from build123d import *

# Parameters (mm, degrees)
BOSS_EXTRUDE1_DEPTH = 8
SKETCH2_R           = 26
SKETCH2_R_2         = 22.5
EXTRUDE_THIN1_DEPTH = 50
SKETCH3_R           = 24.5
SKETCH3_R_2         = 22.5
EXTRUDE_THIN2_DEPTH = 40


with BuildPart() as part:
    # Sketch1 → Boss-Extrude1 (new body)
    with BuildSketch(Plane(origin=(0, 0, 0), x_dir=(1, 0, 0), z_dir=(0, 1, 0))):
        with BuildLine():
            ThreePointArc((-7.74066092, -30.276140252), (0, -31.25), (7.74066092, -30.276140252))
            ThreePointArc((7.74066092, -30.276140252), (32.571933158, -26.108732409), (57.750443262, -26.153431792))
            ThreePointArc((57.750443262, -26.153431792), (86.25, 0), (57.750443262, 26.153431792))
            ThreePointArc((57.750443262, 26.153431792), (32.571933158, 26.108732409), (7.74066092, 30.276140252))
            ThreePointArc((7.74066092, 30.276140252), (0, 31.25), (-7.74066092, 30.276140252))
            ThreePointArc((-7.74066092, 30.276140252), (-32.571933158, 26.108732409), (-57.750443262, 26.153431792))
            ThreePointArc((-57.750443262, 26.153431792), (-86.25, 0), (-57.750443262, -26.153431792))
            ThreePointArc((-57.750443262, -26.153431792), (-32.571933158, -26.108732409), (-7.74066092, -30.276140252))
        make_face()
    extrude(amount=BOSS_EXTRUDE1_DEPTH)

    # Sketch2 → Extrude-Thin1 (add)
    with BuildSketch(Plane(origin=(0, 8, 0), x_dir=(1, 0, 0), z_dir=(0, 1, 0))):
        Circle(SKETCH2_R)
        Circle(SKETCH2_R_2, mode=Mode.SUBTRACT)
    extrude(amount=EXTRUDE_THIN1_DEPTH)

    # Sketch3 → Extrude-Thin2 (add)
    # profile 1 of 2: a face of its own
    with BuildSketch(Plane.XZ):
        with Locations((-60, 0)):
            Circle(SKETCH3_R)
        with Locations((-60, 0)):
            Circle(SKETCH3_R_2, mode=Mode.SUBTRACT)
    # profile 2 of 2: a face of its own
    with BuildSketch(Plane.XZ):
        with Locations((60, 0)):
            Circle(SKETCH3_R)
        with Locations((60, 0)):
            Circle(SKETCH3_R_2, mode=Mode.SUBTRACT)
    extrude(amount=EXTRUDE_THIN2_DEPTH)


solid = part.part
Read the model definition and answer for the solid it produces. Units are mm, in the model's axes. A direction names the side the tool comes from. Round coordinates to 2 decimals unless told otherwise and drop trailing zeros. Loops run counter-clockwise (first coordinate to the right, second up) from the corner with the lowest first, then second, coordinate; pieces in that order, holes last.
Q1. Section C-C on z = -2 is taken. Write down the section's boundary in (x, y), and give its area (3 significant figures).
Q2. Which of the six approach directions +Z, -Z, +X, -X, +Y, -Y give full straight-line access (tool end or side, diameter ignored) to faces 1 (the face through (-60, 0, 0)), 2 (the face through (32.92, 3.94, -26.08)), 3 (the face through (0, 8, 0))?
Q3. Each of these flat-tipped pins is pushed along its axis until it touches: pin 1 (10 mm diameter, centred on x = -4, z = -6.5, fed in from +Y); pin 2 (1 mm diameter, centred on y = 2, z = 8, fed in from +X); pin 3 (1 mm diameter, centred on x = -9.5, z = 23.5, fed in from -Y). Where does it stop, or does it pass through?
Q4. Determine the mould class of faces 4 (the face through (0.11, 3.94, -31.25)), 5 (the face through (10.382, 32.65, 19.961)), 6 (the face through (-32.92, 3.94, 26.08)) for opening direction Z: released by +Z, released by -Z, zero draft, split by the parting line, or undercut.
Q5. Consider probe 1 along X at (y, z) = (-7, 1); probe 2 along X at (y, z) = (39, 0); probe 3 along Z at (x, y) = (60, -17). Determine where each line is inside the solid, lowest interval first.
Q6. Section A-A on y = -8 is taken. Write down the section's boundary in (x, z), and give its area (3 significant figures).
Q7. Section B-B on x = -60 is taken. Write down the section's boundary in (y, z), and give its area (3 significant figures).
Q8. Section D-D on x = 0 is taken. Write down the section's boundary in (y, z), and give its area (3 significant figures).
Output:
1. outline: (-86.17, 0) - (-84.42, 0) - (-84.42, -40) - (-82.41, -40) - (-82.41, 0) - (-37.59, 0) - (-37.59, -40) - (-35.58, -40) - (-35.58, 0) - (35.58, 0) - (35.58, -40) - (37.59, -40) - (37.59, 0) - (82.41, 0) - (82.41, -40) - (84.42, -40) - (84.42, 0) - (86.17, 0) - (86.17, 8) - (25.92, 8) - (25.92, 58) - (22.41, 58) - (22.41, 8) - (-22.41, 8) - (-22.41, 58) - (-25.92, 58) - (-25.92, 8) - (-86.17, 8) - close
1. area: 2,050 mm2
2. face 1: -Y
2. face 2: -Z, +Y, -Y
2. face 3: +Y
3. pin 1: stops at y = 8
3. pin 2: stops at x = 85.16
3. pin 3: stops at y = 0
4. face 4: released by -Z
4. face 5: undercut
4. face 6: released by +Z
5. probe 1: x = -84.48 to -82.48, -37.52 to -35.52, 35.52 to 37.52, 82.48 to 84.48
5. probe 2: x = -26 to -22.5, 22.5 to 26
5. probe 3: z = -24.5 to -22.5, 22.5 to 24.5
6. outline: circle Ø49 at (-60, 0); circle Ø49 at (60, 0); hole circle Ø45 at (-60, 0); hole circle Ø45 at (60, 0)
6. area: 591 mm2
7. outline: (-40, -24.5) - (0, -24.5) - (0, -26.25) - (8, -26.25) - (8, 26.25) - (0, 26.25) - (0, 24.5) - (-40, 24.5) - (-40, 22.5) - (0, 22.5) - (0, -22.5) - (-40, -22.5) - close
7. area: 580 mm2
8. outline: (0, -31.25) - (8, -31.25) - (8, -26) - (58, -26) - (58, -22.5) - (8, -22.5) - (8, 22.5) - (58, 22.5) - (58, 26) - (8, 26) - (8, 31.25) - (0, 31.25) - close
8. area: 850 mm2
